```python
from build123d import *
from OCP.BRepFilletAPI import BRepFilletAPI_MakeChamfer

# Parameters (mm, degrees)
SKETCH1_R             = 5
BOSS_EXTRUDE1_DEPTH   = 5.1
BOSS_EXTRUDE1_2_DEPTH = 5.1
BOSS_EXTRUDE2_DEPTH   = 4
BOSS_EXTRUDE3_DEPTH   = 4
BOSS_EXTRUDE4_DEPTH   = 6
SKETCH5_R             = 3.5
CUT_EXTRUDE1_DEPTH    = 57.105347339
SKETCH7_R             = 2.75
CUT_EXTRUDE2_DEPTH    = 41.851070977
BOSS_EXTRUDE5_DEPTH   = 14
FILLET1_R             = 4
FILLET2_R             = 4
FILLET3_R             = 4
CHAMFER1_SIZE         = 1
CHAMFER1_SIZE2        = 0.577350269


with BuildPart() as part:
    # Sketch1 → Boss-Extrude1 (new body)
    with BuildSketch(Plane(origin=(0, 0, 0), x_dir=(0, 0, -1), z_dir=(1, 0, 0))):
        with Locations((30, 0)):
            Circle(SKETCH1_R)
    extrude(amount=BOSS_EXTRUDE1_DEPTH)



with BuildPart() as body_2:
    # Sketch1 → Boss-Extrude1 2 (new body)
    with BuildSketch(Plane(origin=(0, 0, 0), x_dir=(0, 0, -1), z_dir=(1, 0, 0))):
        with Locations((-30, 0)):
            Circle(SKETCH1_R)
    extrude(amount=BOSS_EXTRUDE1_2_DEPTH)


with BuildPart() as part_1:
    add(part.part)

    add(body_2.part)  # Boss-Extrude2 merges body 2
    # Sketch2 → Boss-Extrude2 (add)
    with BuildSketch(Plane(origin=(5.1, 0, 0), x_dir=(0, 0, -1), z_dir=(1, 0, 0))):
        with BuildLine():
            Line((30, -5), (-30, -5))
            ThreePointArc((-30, -5), (-33.535533906, -3.535533906), (-35, 0))
            Line((-35, 0), (-35, 5))
            Line((-35, 5), (-35, 9))
            Line((-35, 9), (35, 9))
            Line((35, 9), (35, 0))
            ThreePointArc((35, 0), (33.535533906, -3.535533906), (30, -5))
        make_face()
    extrude(amount=BOSS_EXTRUDE2_DEPTH)

    # Sketch3 → Boss-Extrude3 (add)
    with BuildSketch(Plane(origin=(0, 9, 0), x_dir=(1, 0, 0), z_dir=(0, 1, 0))):
        Polygon((5.1, 17), (-4.9, 17), (-6.4, 17), (-6.4, 3), (-4.9, 3), (9.1, 3), (9.1, 17), align=None)
    extrude(amount=BOSS_EXTRUDE3_DEPTH)

    # Sketch4 → Boss-Extrude4 (add)
    with BuildSketch(Plane(origin=(0, 13, 0), x_dir=(1, 0, 0), z_dir=(0, 1, 0))):
        Polygon((3.1, 17), (-6.4, 17), (-6.4, 3), (3.1, 3), (3.1, 10), align=None)
    extrude(amount=BOSS_EXTRUDE4_DEPTH)

    # Sketch5 → Cut-Extrude1 (cut, through all)
    with BuildSketch(Plane.XY.offset(-17)):
        with Locations(Location((-1.5, 14, 0), (0, 0, 180))):
            Circle(SKETCH5_R)
    extrude(amount=CUT_EXTRUDE1_DEPTH, mode=Mode.SUBTRACT)

    # Sketch7 → Cut-Extrude2 (cut, through all)
    with BuildSketch(Plane.ZY):
        with Locations((-30, 0)):
            Circle(SKETCH7_R)
        with Locations((30, 0)):
            Circle(SKETCH7_R)
    extrude(amount=-CUT_EXTRUDE2_DEPTH, mode=Mode.SUBTRACT)

    # Sketch8 → Boss-Extrude5 (add)
    with BuildSketch(Plane(origin=(0, 0, -17), x_dir=(-1, 0, 0), z_dir=(0, 0, -1))):
        Polygon((-9.1, 13), (-3.1, 19), (-3.1, 13), align=None)
    extrude(amount=-BOSS_EXTRUDE5_DEPTH)

    # Fillet1
    fillet1_edges = [part_1.edges().sort_by_distance(p)[0] for p in [
        (-6.4, 9, -10),
        (-6.4, 19, -10),
        (3.1, 19, -10),
    ]]
    fillet(fillet1_edges, radius=FILLET1_R - 0.0001)  # a hair under: the kernel refuses the full size

    # Fillet2
    fillet2_edges = [part_1.edges().sort_by_distance(p)[0] for p in [
        (7.1, 9, -3),
        (7.1, 9, -17),
    ]]
    fillet(fillet2_edges, radius=FILLET2_R)

    # Fillet3
    fillet3_edges = [part_1.edges().sort_by_distance(p)[0] for p in [
        (7.1, 9, -35),
        (7.1, 9, 35),
    ]]
    fillet(fillet3_edges, radius=FILLET3_R)

    # Chamfer1: one chamfer whose edges measure the first distance from different faces: ONE call of the kernel's chamfer builder (chamfer() names one face for all edges)
    chamfer1_edges_1 = [part_1.edges().sort_by_distance(p)[0] for p in [
        (0, 0, -25),
    ]]
    chamfer1_side_1 = [part_1.faces().sort_by_distance(p)[0] for p in [
        (0, 0, -25.141421356),
    ]]
    chamfer1_edges_2 = [part_1.edges().sort_by_distance(p)[0] for p in [
        (0, 0, 35),
    ]]
    chamfer1_side_2 = [part_1.faces().sort_by_distance(p)[0] for p in [
        (0, 0, 34.858578644),
    ]]
    chamfer1 = BRepFilletAPI_MakeChamfer(part_1.part.solid().wrapped)
    for e in chamfer1_edges_1:
        chamfer1.Add(CHAMFER1_SIZE, CHAMFER1_SIZE2, e.wrapped, chamfer1_side_1[0].wrapped)  # the first distance lies on this face
    for e in chamfer1_edges_2:
        chamfer1.Add(CHAMFER1_SIZE, CHAMFER1_SIZE2, e.wrapped, chamfer1_side_2[0].wrapped)  # the first distance lies on this face
    add(Compound.cast(chamfer1.Shape()), mode=Mode.REPLACE)


solid = part_1.part
```
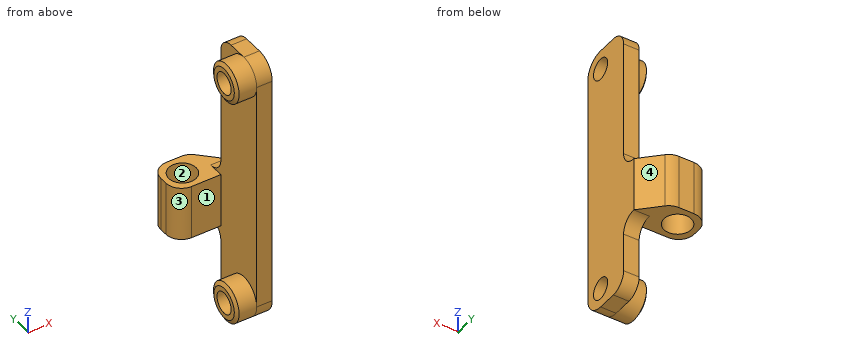
Could you check a few things on this model? Use its own coordinates, in mm. Face numbers are marked on the shaded views. Coordinates: 2 decimals unless noted, no trailing zeros. Order: outer loops, then holes, each group sorted by start corner. A loop starts at its lowest first (then second) coordinate and runs counter-clockwise, first axis right, second up. Notation, with made-up numbers: M -16,55.5 L 43,55.5 A16 cw 43,60.5 Z; hole C 25,17 d9. An arc over 180 degrees is marked long. Use one line per item in the form item = value. Start each with the question number.
1. Suppose I cut it at B-B on x = -1.5. Write out the boundary of the cut face in (y, z), then the cut area to 3 significant figures.
2. For pin 1 (3 mm diameter, centred on x = -2, z = 27, fed in from +Y); pin 2 (2 mm diameter, centred on y = 8.5, z = 22, fed in from -X); pin 3 (6 mm diameter, centred on x = 0.5, z = -11, fed in from -Y); pin 4 (9 mm diameter, centred on y = 0.5, z = 32, fed in from -X), each with a flat end and sliding along its axis, tell me the tip position at first contact or that it passes through.
3. We'd pull the mould along X, two halves only. Please class the marked faces 1, 2, 3 and 4: +X half, -X half, draft (parallel to the pull), parting line (faces both ways), or undercut.
4. Suppose I cut it at A-A on z = -13. Write out the boundary of the cut face in (x, y), then the cut area to 3 significant figures.
5. Suppose I cut it at D-D on x = 7.25. Write out the boundary of the cut face in (y, z).
6. Suppose I cut it at C-C on y = 14. Write out the boundary of the cut face in (x, z).
7. Please list where these lines run through material, in increasing order: line 1 (Y direction, x = 6.25, z = 30); line 2 (Y direction, x = 3.25, z = -30); line 3 (Z direction, x = 5.75, y = 2).
Geometry says:
q1.outline = M 9,-17 L 10.5,-17 L 10.5,-3 L 9,-3 Z; M 17.5,-17 L 19,-17 L 19,-3 L 17.5,-3 Z
q1.area = 42.0 mm^2
q2.pin_1 = through
q2.pin_2 = 5.1
q2.pin_3 = 9
q2.pin_4 = 0
q3.face_1 = draft
q3.face_2 = undercut
q3.face_3 = -X half
q3.face_4 = +X half
q4.outline = M -6.4,13 A4 ccw -2.4,9 L 5.1,9 L 5.1,-5 L 9.1,-5 L 9.1,13 L 4.27,17.83 A4 ccw 1.44,19 L -2.4,19 A4 ccw -6.4,15 Z; hole C -1.5,14 d7
q4.area = 147 mm^2
q5.outline = M -5,-30 A5 ccw 0,-35 L 5,-35 A4 ccw 9,-31 L 9,-21 A4 cw 13,-17 L 14.85,-17 L 14.85,-3 L 13,-3 A4 cw 9,1 L 9,31 A4 ccw 5,35 L 0,35 A5 ccw -5,30 Z; hole C 0,-30 d5.5; hole C 0,30 d5.5
q6.outline = M -6.4,-17 L -5,-17 L -5,-3 L -6.4,-3 Z; M 2,-17 L 8.1,-17 L 8.1,-3 L 2,-3 Z
q7.line_1 = -5 to -2.75, 2.75 to 9
q7.line_2 = -5 to -2.75, 2.75 to 5
q7.line_3 = -35 to -31.89, -28.11 to 28.11, 31.89 to 35
